from build123d import *

# Parameters (mm, degrees)
SZKIC1_W                    = 42.3
SZKIC1_H                    = 42.3
DODANIE_WYCI_GNI_CIE1_DEPTH = 22
SFAZOWANIE1_SIZE            = 7
ZAOKR_GLENIE1_R             = 3
WYTNIJ_WYCI_GNI_CIE1_REACH  = 39.13
SZKIC2_R                    = 20
SZKIC2_R_2                  = 1.75


with BuildPart() as part:
    # Szkic1 → Dodanie-wyciągnięcie1 (new body)
    with BuildSketch(Plane.XY):
        Rectangle(SZKIC1_W, SZKIC1_H)
    extrude(amount=DODANIE_WYCI_GNI_CIE1_DEPTH)

    # Sfazowanie1
    sfazowanie1_edges = [part.edges().sort_by_distance(p)[0] for p in [
        (21.15, -21.15, 11),
        (-21.15, -21.15, 11),
        (-21.15, 21.15, 11),
        (21.15, 21.15, 11),
    ]]
    chamfer(sfazowanie1_edges, length=SFAZOWANIE1_SIZE)

    # Zaokrąglenie1
    zaokr_glenie1_edges = [part.edges().sort_by_distance(p)[0] for p in [
        (14.15, -21.15, 11),
        (-14.15, -21.15, 11),
        (-21.15, 14.15, 11),
        (-21.15, -14.15, 11),
        (21.15, 14.15, 11),
        (21.15, -14.15, 11),
        (14.15, 21.15, 11),
        (-14.15, 21.15, 11),
    ]]
    fillet(zaokr_glenie1_edges, radius=ZAOKR_GLENIE1_R)

    # Szkic2 → Wytnij-wyciągnięcie1 (cut, up to next)
    with BuildSketch(Plane.XY.offset(22), mode=Mode.PRIVATE) as wytnij_wyci_gni_cie1_sk1:
        Circle(SZKIC2_R)
    wytnij_wyci_gni_cie1_tool1 = extrude(wytnij_wyci_gni_cie1_sk1.sketch, amount=-WYTNIJ_WYCI_GNI_CIE1_REACH, mode=Mode.PRIVATE) & part.part
    # Szkic2 → Wytnij-wyciągnięcie1 (cut, up to next)
    with BuildSketch(Plane.XY.offset(22), mode=Mode.PRIVATE) as wytnij_wyci_gni_cie1_sk2:
        with Locations((-15.5, 15.5)):
            Circle(SZKIC2_R_2)
    wytnij_wyci_gni_cie1_tool2 = extrude(wytnij_wyci_gni_cie1_sk2.sketch, amount=-WYTNIJ_WYCI_GNI_CIE1_REACH, mode=Mode.PRIVATE) & part.part
    # Szkic2 → Wytnij-wyciągnięcie1 (cut, up to next)
    with BuildSketch(Plane.XY.offset(22), mode=Mode.PRIVATE) as wytnij_wyci_gni_cie1_sk3:
        with Locations((15.5, 15.5)):
            Circle(SZKIC2_R_2)
    wytnij_wyci_gni_cie1_tool3 = extrude(wytnij_wyci_gni_cie1_sk3.sketch, amount=-WYTNIJ_WYCI_GNI_CIE1_REACH, mode=Mode.PRIVATE) & part.part
    # Szkic2 → Wytnij-wyciągnięcie1 (cut, up to next)
    with BuildSketch(Plane.XY.offset(22), mode=Mode.PRIVATE) as wytnij_wyci_gni_cie1_sk4:
        with Locations((15.5, -15.5)):
            Circle(SZKIC2_R_2)
    wytnij_wyci_gni_cie1_tool4 = extrude(wytnij_wyci_gni_cie1_sk4.sketch, amount=-WYTNIJ_WYCI_GNI_CIE1_REACH, mode=Mode.PRIVATE) & part.part
    # Szkic2 → Wytnij-wyciągnięcie1 (cut, up to next)
    with BuildSketch(Plane.XY.offset(22), mode=Mode.PRIVATE) as wytnij_wyci_gni_cie1_sk5:
        with Locations((-15.5, -15.5)):
            Circle(SZKIC2_R_2)
    wytnij_wyci_gni_cie1_tool5 = extrude(wytnij_wyci_gni_cie1_sk5.sketch, amount=-WYTNIJ_WYCI_GNI_CIE1_REACH, mode=Mode.PRIVATE) & part.part
    add(wytnij_wyci_gni_cie1_tool1.solids().sort_by_distance((0, 0, 22))[0], mode=Mode.SUBTRACT)
    add(wytnij_wyci_gni_cie1_tool2.solids().sort_by_distance((-15.5, 15.5, 22))[0], mode=Mode.SUBTRACT)
    add(wytnij_wyci_gni_cie1_tool3.solids().sort_by_distance((15.5, 15.5, 22))[0], mode=Mode.SUBTRACT)
    add(wytnij_wyci_gni_cie1_tool4.solids().sort_by_distance((15.5, -15.5, 22))[0], mode=Mode.SUBTRACT)
    add(wytnij_wyci_gni_cie1_tool5.solids().sort_by_distance((-15.5, -15.5, 22))[0], mode=Mode.SUBTRACT)


solid = part.part
Here's how the part is built. I have some questions about the finished solid (model axes, mm). Coordinates: 2 decimals unless noted, no trailing zeros. Write each loop counter-clockwise with the first axis right and the second up, starting at its lowest first coordinate (ties: lowest second). Pieces come first, ordered by that corner, then holes.
1) If we section it at C-C (z = 5.25): List the corners of the cut face in (x, y) for me.
Filled in:
outline: (-21.15, -12.91) arc R3 ccw to (-20.27, -15.03) - (-15.03, -20.27) arc R3 ccw to (-12.91, -21.15) - (12.91, -21.15) arc R3 ccw to (15.03, -20.27) - (20.27, -15.03) arc R3 ccw to (21.15, -12.91) - (21.15, 12.91) arc R3 ccw to (20.27, 15.03) - (15.03, 20.27) arc R3 ccw to (12.91, 21.15) - (-12.91, 21.15) arc R3 ccw to (-15.03, 20.27) - (-20.27, 15.03) arc R3 ccw to (-21.15, 12.91) - close; hole circle Ø40 at (0, 0); hole circle Ø3.5 at (-15.5, -15.5); hole circle Ø3.5 at (-15.5, 15.5); hole circle Ø3.5 at (15.5, -15.5); hole circle Ø3.5 at (15.5, 15.5)
2) I'm going to push a flat-ended pin straight in: pin 1 (12 mm diameter, centred on x = 7.5, y = 10.5, fed in from -Z). Where does the tip first touch, or does it pass through?
Filled in:
pin 1: passes through
3) If we section it at A-A (x = 0): List the corners of the cut face in (y, z) for me, plus the area to 3 significant figures.
Filled in:
outline: (-21.15, 0) - (-20, 0) - (-20, 22) - (-21.15, 22) - close; (20, 0) - (21.15, 0) - (21.15, 22) - (20, 22) - close
area: 50.6 mm2
4) If we section it at D-D (y = -14.5): List the corners of the cut face in (x, z) for me.
Filled in:
outline: (-20.69, 0) - (-16.94, 0) - (-16.94, 22) - (-20.69, 22) - close; (-14.06, 0) - (-13.77, 0) - (-13.77, 22) - (-14.06, 22) - close; (13.77, 0) - (14.06, 0) - (14.06, 22) - (13.77, 22) - close; (16.94, 0) - (20.69, 0) - (20.69, 22) - (16.94, 22) - close
5) If I drill on line 1 (Y direction, x = 0, z = 17); line 2 (Y direction, x = 17, z = 20); line 3 (Y direction, x = 15.5, z = 13), over which ranges is the centre line in solid material (lowest first)?
Filled in:
line 1: y = -21.15 to -20, 20 to 21.15
line 2: y = -18.3 to -16.4, -14.6 to -10.54, 10.54 to 14.6, 16.4 to 18.3
line 3: y = -19.8 to -17.25, -13.75 to -12.64, 12.64 to 13.75, 17.25 to 19.8
6) Thinking about a two-plate mould opening in Y: for faces 1 (the face through (20.915, 14.071, 11.154)), 2 (the face through (17.7, -17.6, 10.8)), 3 (the face through (15.272, 17.235, 11.154)), 4 (the face through (-14.6, -14, 11.2)), which applies, +Y half, -Y half, draft (parallel to the pull), parting line (faces both ways), or undercut?
Filled in:
face 1: +Y half
face 2: -Y half
face 3: undercut
face 4: undercut
